Build history of the part. All positions in model axes, mm. Coordinates: 2 decimals unless noted, no trailing zeros. Loops run counter-clockwise (first coordinate to the right, second up) from the corner with the lowest first, then second, coordinate; pieces in that order, holes last. Notation, with made-up numbers: M 20,73.5 L 50,73.5 A11 cw 50,91.5 Z; hole C 83,-1.5 d7. An arc over 180 degrees is marked long. Write each question's results on one line, items separated by ' | '. Start each with the question number.
from build123d import *

# Parameters (mm, degrees)
F0_W     = 288
F0_H     = 177
F0_R     = 2
F0_W_2   = 258
F0_H_2   = 138
F1_DEPTH = 3
F2_R     = 5


with BuildPart() as f1:
    # F0 (on Top) → F1 (new body)
    with BuildSketch(Plane.XY):
        with Locations((0, 7.5)):
            Rectangle(F0_W, F0_H)
        with Locations((-84, -76)):
            Circle(F0_R, mode=Mode.SUBTRACT)
        with Locations((-69, -76)):
            Circle(F0_R, mode=Mode.SUBTRACT)
        with Locations((69, -76)):
            Circle(F0_R, mode=Mode.SUBTRACT)
        with Locations((84, -76)):
            Circle(F0_R, mode=Mode.SUBTRACT)
        with Locations((-139, 46)):
            Circle(F0_R, mode=Mode.SUBTRACT)
        with Locations((-94, 91)):
            Circle(F0_R, mode=Mode.SUBTRACT)
        with Locations((0, 14)):
            Rectangle(F0_W_2, F0_H_2, mode=Mode.SUBTRACT)
        with Locations((139, 46)):
            Circle(F0_R, mode=Mode.SUBTRACT)
        with Locations((94, 91)):
            Circle(F0_R, mode=Mode.SUBTRACT)
    extrude(amount=F1_DEPTH)

    # F2
    f2_edges = [f1.edges().sort_by_distance(p)[0] for p in [
        (-144, 96, 1.5),
        (-144, -81, 1.5),
        (144, -81, 1.5),
        (144, 96, 1.5),
    ]]
    fillet(f2_edges, radius=F2_R)


solid = f1.part
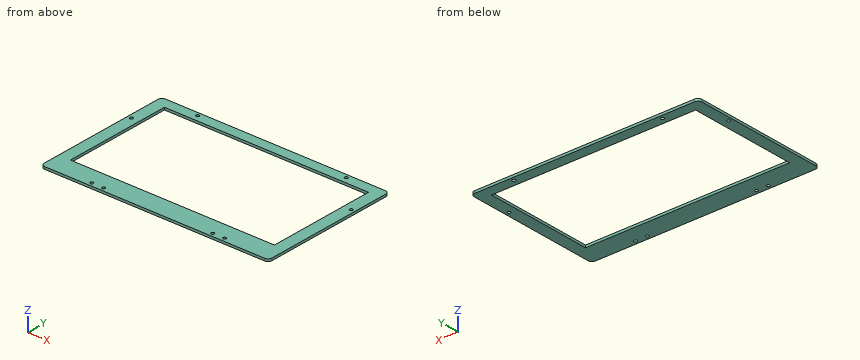
1. Pin check, flat tip, straight feed: pin 1 (3 mm diameter, centred on x = 84, y = -76, fed in from -Z). Stop position of the tip, or through.
2. Wall check: line 1 along Y through (x, z) = (69, 2); line 2 along X through (y, z) = (-5, 1); line 3 along Y through (x, z) = (14.5, 1.15). Give the ranges that are in metal, low to high.
3. Band-saw the part on B-B, the plane z = 0.6. Give the number of separate pieces and of enclosed holes in the cut face, plus the area to 4 significant figures.
4. Band-saw the part on C-C, the plane y = -24. List the corners of the cut face in (x, z).
5. Band-saw the part on A-A, the plane x = 56.5. List the corners of the cut face in (y, z).
Checked values:
1) pin 1: through
2) line 1: -81 to -78, -74 to -55, 83 to 96 | line 2: -144 to -129, 129 to 144 | line 3: -81 to -55, 83 to 96
3) separate pieces: 1 | enclosed holes: 9 | area: 15,250 mm²
4) outline: M -144,0 L -129,0 L -129,3 L -144,3 Z; M 129,0 L 144,0 L 144,3 L 129,3 Z
5) outline: M -81,0 L -55,0 L -55,3 L -81,3 Z; M 83,0 L 96,0 L 96,3 L 83,3 Z
